```python
from build123d import *

# Parameters (mm, degrees)
CHAMFER2_SIZE = 0.5


with BuildPart() as part:
    # Sketch4 → Revolve1 (revolve)
    with BuildSketch(Plane.XY):
        Polygon((-1, 0), (-1, 26.5), (-3, 26.5), (-3, 8.6), (-2, 7.6), (-2, 6), (-3, 5), (-3, 0), align=None)
    revolve(axis=Axis((0, -1000, 0), (0, 1, 0)))

    # Chamfer2
    chamfer2_edges = [part.edges().sort_by_distance(p)[0] for p in [
        (3, 0, 0),
        (3, 26.5, 0),
        (1, 26.5, 0),
    ]]
    chamfer(chamfer2_edges, length=CHAMFER2_SIZE)


solid = part.part
```
Geometry check sheet. Reference: the model listing, model coordinates, mm. Coordinates: 2 decimals unless noted, no trailing zeros. Write each loop counter-clockwise with the first axis right and the second up, starting at its lowest first coordinate (ties: lowest second). Pieces come first, ordered by that corner, then holes. Notation, with made-up numbers: M -15,-39 L 24,-39 A20 ccw 24,-2 Z; hole C 37,48.5 d8. An arc over 180 degrees is marked long. Use one line per item in the form item = value. Start each with the question number.
1) Section check B-B on x = 0. Enter the section's corners in (y, z), and give its area (3 significant figures).
2) Section check A-A on z = 0. Enter the section's corners in (x, y), and give its area (3 significant figures).
3) Thickness scan on probe 1 along Z at (x, y) = (0, 11.75); probe 2 along Y at (x, z) = (2.3, -1.4); probe 3 along Y at (x, z) = (-1.5, -1.6). Record the ranges inside material, lowest first. Write a range as from..to.
4) Section check C-C on y = 19. Enter the section's corners in (x, z).
5) Release check for a two-part mould opening along Y. For faces 1 (the cylindrical face through (3, 3, 0)), 2 (the cylindrical face through (0, 7, -2)), 3 (the flat face through (2, 26.5, 0)) record: pulls with the +Y half, pulls with the -Y half, needs draft (parallel to the pull), parting line crosses it, or undercut.
6) Go/stop test with flat-tipped pins: pin 1 Ø2 at (y, z) = (17.5, -2.5) entering from +X; pin 2 Ø2 at (y, z) = (13, -1.5) entering from -X. Record where each tip stops, or that it passes through.
Responses:
q1.outline = M 0,-2.5 L 0.5,-3 L 5,-3 L 6,-2 L 7.6,-2 L 8.6,-3 L 26,-3 L 26.5,-2.5 L 26.5,-1.5 L 26,-1 L 0,-1 Z; M 0,1 L 26,1 L 26.5,1.5 L 26.5,2.5 L 26,3 L 8.6,3 L 7.6,2 L 6,2 L 5,3 L 0.5,3 L 0,2.5 Z
q1.area = 100 mm2
q2.outline = M -3,0.5 L -2.5,0 L -1,0 L -1,26 L -1.5,26.5 L -2.5,26.5 L -3,26 L -3,8.6 L -2,7.6 L -2,6 L -3,5 Z; M 1,0 L 2.5,0 L 3,0.5 L 3,5 L 2,6 L 2,7.6 L 3,8.6 L 3,26 L 2.5,26.5 L 1.5,26.5 L 1,26 Z
q2.area = 100 mm2
q3.probe_1 = -3..-1, 1..3
q3.probe_2 = 0.19..5.31, 8.29..26.31
q3.probe_3 = 0..5.81, 7.79..26.5
q4.outline = C 0,0 d6; hole C 0,0 d2
q5.face_1 = needs draft
q5.face_2 = undercut
q5.face_3 = pulls with the +Y half
q6.pin_1 = 2.6
q6.pin_2 = -2.96
